For this review, take the finished solid that the model builds, in its own axes (mm). Face numbers are marked on the shaded views. A direction names the side the tool comes from. Round coordinates to 2 decimals unless told otherwise and drop trailing zeros. Write each loop counter-clockwise with the first axis right and the second up, starting at its lowest first coordinate (ties: lowest second). Pieces come first, ordered by that corner, then holes. Notation, with made-up numbers: (66.5, -5.75) -> (72.5, -5.75) arc R25 ccw to (72.5, 13.25) -> close; hole circle Ø9 at (-13, 5). An arc over 180 degrees is marked (long way). Answer in a Markdown table with one row per item. Add a question column.
Autodesk Inventor part; units mm, degrees
ref_plane "YZ Plane" through (0, 0, 0) normal (1, 0, 0) x (0, 1, 0)
ref_plane "XZ Plane" through (0, 0, 0) normal (0, 1, 0) x (-1, 0, 0)
ref_plane "XY Plane" through (0, 0, 0) normal (0, 0, 1) x (1, 0, 0)
sketch "Sketch1" plane through (0, 0, 0) normal (0, 0, 1) x (1, 0, 0)
  line L0 (-37.8857, 18.2857) -> (-32.9327, 18.2857)
  line L1 (-32.9327, 18.2857) -> (-32.9327, 15.8981)
  line L2 (-32.9327, 15.8981) -> (-37.8857, 15.8981)
  line L3 (-37.8857, 15.8981) -> (-37.8857, 18.2857)
  dimension "d0" = 4.953
  dimension "d1" = 2.3876
extrude "Extrusion1" add sketch "Sketch1" along normal blind 7.62
sketch "Sketch2" plane through (-37.8857, 15.8981, 0) normal (0, -1, 0) x (1, 0, 0)
  line L0 (4.953, 7.62) -> (0, 7.62)
  line L1 (1.6764, 7.62) -> (3.2766, 7.62)
  line L2 (3.2766, 7.62) -> (3.2766, 6.35)
  line L3 (3.2766, 6.35) -> (1.6764, 6.35)
  line L4 (1.6764, 6.35) -> (1.6764, 7.62)
  line L5 (0, 0) -> (0, 7.62)
  line L6 (4.953, 0) -> (4.953, 7.62)
  line L7 (4.953, 7.0612) -> (4.191, 7.0612)
  line L8 (4.191, 7.0612) -> (4.191, 6.35)
  line L9 (4.191, 6.35) -> (4.953, 6.35)
  line L10 (4.953, 6.35) -> (4.953, 7.0612)
  line L11 (0, 12.9286) -> (0.762, 12.9286)
  line L12 (0.762, 12.9286) -> (0.762, 12.2174)
  line L13 (0.762, 12.2174) -> (0, 12.2174)
  line L14 (0, 12.2174) -> (0, 12.9286)
  dimension "d4" = 1.6764
  dimension "d5" = 1.6764
  dimension "d6" = 1.27
  dimension "d9" = 0.5588
  dimension "d12" = 0
  dimension "d13" = 0.762
  dimension "d14" = 0.762
extrude "Extrusion2" cut sketch "Sketch2" against normal blind 13.4874
sketch "Sketch3" plane through (-33.6947, 15.8981, 7.0612) normal (1, 0, 0) x (0, 0, -1)
  line L0 (0, 2.3876) -> (0.7112, 2.3876)
  line L1 (0.7112, 0) -> (0, 0)
  line L2 (0.7112, 0) -> (0.7112, 2.3876)
  line L3 (0, 2.3876) -> (0.7112, 2.3876)
  line L4 (0.7112, 2.3876) -> (0.7112, 2.0066)
  line L5 (0.7112, 2.0066) -> (0, 2.0066)
  line L6 (0, 2.0066) -> (0, 2.3876)
  line L7 (0, 0) -> (0.7112, 0)
  line L8 (0.7112, 0) -> (0.7112, 0.381)
  line L9 (0.7112, 0.381) -> (0, 0.381)
  line L10 (0, 0.381) -> (0, 0)
  dimension "d15" = 0.381
  dimension "d16" = 0.381
extrude "Extrusion3" cut sketch "Sketch3" against normal blind 13.4874
sketch "Sketch4" plane through (0, 0, 7.62) normal (0, 0, 1) x (1, 0, 0)
  line L0 (-36.2093, 15.8981) -> (-36.2093, 18.2857)
  line L1 (-37.8857, 18.2857) -> (-36.2093, 18.2857)
  line L2 (-36.2093, 15.8981) -> (-37.8857, 15.8981)
  line L3 (-36.2093, 17.3205) -> (-36.6665, 17.3205)
  line L4 (-36.6665, 17.3205) -> (-36.6665, 16.8633)
  line L5 (-36.6665, 16.8633) -> (-36.2093, 16.8633)
  line L6 (-36.2093, 16.8633) -> (-36.2093, 17.3205)
  line L7 (-34.6091, 18.2857) -> (-34.6091, 15.8981)
  line L8 (-32.9327, 15.8981) -> (-34.6091, 15.8981)
  line L9 (-32.9327, 18.2857) -> (-32.9327, 15.8981)
  line L10 (-34.6091, 18.2857) -> (-32.9327, 18.2857)
  line L11 (-34.6091, 17.3205) -> (-34.1519, 17.3205)
  line L12 (-34.1519, 17.3205) -> (-34.1519, 16.8633)
  line L13 (-34.1519, 16.8633) -> (-34.6091, 16.8633)
  line L14 (-34.6091, 16.8633) -> (-34.6091, 17.3205)
  dimension "d19" = 0.4572
  dimension "d20" = 0.4572
  dimension "d21" = 0.4572
  dimension "d22" = 0.4572
  dimension "d23" = 0.9652
  dimension "d24" = 0.9652
  dimension "d25" = 0.9652
extrude "Extrusion4" add sketch "Sketch4" against normal mid plane 0.127 contours L5 L4 L3 L0 | L11 L12 L13 L7
sketch "Sketch5" plane through (-37.8857, 15.8981, 6.35) normal (0, 0, 1) x (1, 0, 0)
  line L0 (3.2766, 0.381) -> (3.2766, 2.0066)
  line L1 (1.6764, 1.4224) -> (1.6764, 0.9652)
  line L2 (1.2192, 1.4224) -> (1.6764, 1.4224)
  line L3 (1.2192, 0.9652) -> (1.2192, 1.4224)
  line L4 (1.6764, 0.9652) -> (1.2192, 0.9652)
  line L5 (3.2766, 1.4224) -> (3.7338, 1.4224)
  line L6 (3.2766, 0.9652) -> (3.2766, 1.4224)
  line L7 (3.7338, 0.9652) -> (3.2766, 0.9652)
  line L8 (3.7338, 1.4224) -> (3.7338, 0.9652)
  line L9 (1.6764, 1.4224) -> (3.2766, 1.4224)
  line L10 (3.2766, 1.4224) -> (3.2766, 1.3261)
  line L11 (3.2766, 1.3261) -> (1.6764, 1.3261)
  line L12 (1.6764, 1.3261) -> (1.6764, 1.4224)
extrude "Extrusion5" add sketch "Sketch5" along normal blind 1.3335 contours L11 L1 L9 L0
equation "\"d5\" = d4"
equation "\"d14\" = d13"
equation "\"d16\" = d15"
equation "\"d20\" = d19"
equation "\"d21\" = d20"
equation "\"d22\" = d21"
equation "\"d24\" = d23"
properties part number "2009_CTS_CopperPost2"
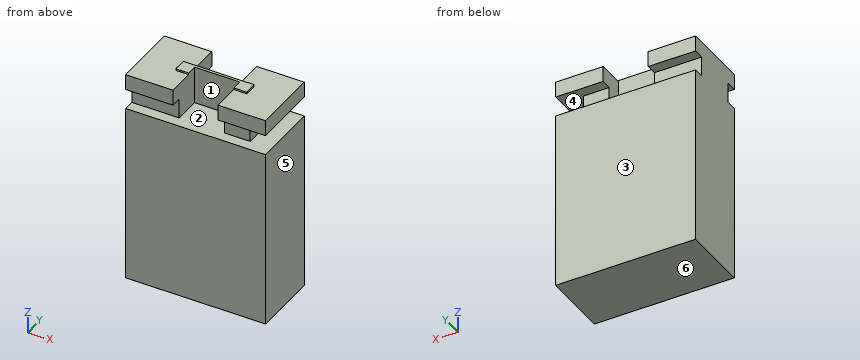
1. We need section B-B (x = -33.35). Write out the cut boundary in (y, z).
2. We need section C-C (z = 7.25). Write out the cut boundary in (x, y), plus the area to 3 significant figures.
3. The part is to be moulded in two halves that separate along Z. For the marked faces 4, 5 and 6, say which applies: pulls with the +Z half, pulls with the -Z half, needs draft (parallel to the pull), parting line crosses it, or undercut.
4. We need section A-A (y = 18.1). Write out the cut boundary in (x, z), plus the area to 3 significant figures.
5. We need section D-D (y = 17.4). Write out the cut boundary in (x, z), plus the area to 3 significant figures.
6. For L1, parallel to Z at x = -37, y = 18.2; L2, parallel to Z at x = -37.1, y = 17.25; L3, parallel to Z at x = -34.9, y = 16.55, list the stretches that pass through material, from the lowest coordinate up. Write a range as [from, to].
7. Tool access review of the marked faces 1, 2 and 3: name each direction out of +Z, -Z, +X, -X, +Y, -Y from which nothing blocks a thin tool from reaching the whole face with its end or side.
8. Clearance check with flat-ended pins moving along their axes: pin 1 Ø0.7 at (x, z) = (-35.5, 7.5) entering from -Y; pin 2 Ø0.5 at (x, y) = (-37, 17) entering from +Z. State where each tip first meets the part, or that it passes through.
Response:
| question | item | result |
|---|---|---|
| 1 | outline | (15.9, 0) -> (18.29, 0) -> (18.29, 6.35) -> (15.9, 6.35) -> close; (15.9, 7.06) -> (18.29, 7.06) -> (18.29, 7.62) -> (15.9, 7.62) -> close |
| 2 | outline | (-37.89, 15.9) -> (-36.21, 15.9) -> (-36.21, 17.22) -> (-34.61, 17.22) -> (-34.61, 15.9) -> (-32.93, 15.9) -> (-32.93, 18.29) -> (-34.61, 18.29) -> (-34.61, 17.32) -> (-36.21, 17.32) -> (-36.21, 18.29) -> (-37.89, 18.29) -> close |
| 2 | area | 8.16 mm2 |
| 3 | face 4 | undercut |
| 3 | face 5 | needs draft |
| 3 | face 6 | pulls with the -Z half |
| 4 | outline | (-37.89, 0) -> (-32.93, 0) -> (-32.93, 6.35) -> (-37.89, 6.35) -> close; (-37.89, 7.06) -> (-36.21, 7.06) -> (-36.21, 7.62) -> (-37.89, 7.62) -> close; (-34.61, 7.06) -> (-32.93, 7.06) -> (-32.93, 7.62) -> (-34.61, 7.62) -> close |
| 4 | area | 33.3 mm2 |
| 5 | outline | (-37.89, 0) -> (-32.93, 0) -> (-32.93, 6.35) -> (-33.69, 6.35) -> (-33.69, 7.06) -> (-32.93, 7.06) -> (-32.93, 7.62) -> (-34.61, 7.62) -> (-34.61, 6.35) -> (-36.21, 6.35) -> (-36.21, 7.62) -> (-37.89, 7.62) -> close |
| 5 | area | 35.2 mm2 |
| 6 | L1 | [0, 6.35], [7.06, 7.62] |
| 6 | L2 | [0, 7.62] |
| 6 | L3 | [0, 6.35] |
| 7 | face 1 | +Z, -Y |
| 7 | face 2 | none |
| 7 | face 3 | +Z, -Z, +X, -X, +Y |
| 8 | pin 1 | y = 17.22 |
| 8 | pin 2 | z = 7.62 |
